The listing builds one solid part. Answer for the finished solid, in the listing's coordinates (mm). Round coordinates to 2 decimals unless told otherwise and drop trailing zeros. Write each loop counter-clockwise with the first axis right and the second up, starting at its lowest first coordinate (ties: lowest second). Pieces come first, ordered by that corner, then holes.
(1) A cutting plane is placed at D-D, the plane x = -80. Give the vertices of the cut face in (y, z).
(2) A cutting plane is placed at A-A, the plane z = 0. Give the vertices of the cut face in (x, y), and give its area (3 significant figures).
(3) Find the intervals of material crossed by probe 1 along Z at (x, y) = (0, -6.5); probe 2 along X at (y, z) = (-7.75, -40); probe 3 along Z at (x, y) = (-40, -4), in increasing order.
(4) This flat-tipped pin is pushed along its axis until it touches: pin 1 Ø10.5 at (x, z) = (-80, 0) entering from +Y. Where does it stop, or does it pass through?
(5) A cutting plane is placed at C-C, the plane z = 40. Give the vertices of the cut face in (x, y).
(6) A cutting plane is placed at B-B, the plane x = 0. Give the vertices of the cut face in (y, z), and give its area (3 significant figures).
from build123d import *

# Parameters (mm, degrees)
BASE_FLANGE1_START     = -75
BASE_FLANGE1_OUTLINE_W = 300
BASE_FLANGE1_OUTLINE_H = 12.7
BASE_FLANGE1_DEPTH     = 150
M10_CLEARANCE_HOLE1_D  = 11
M8_CLEARANCE_HOLE1_D   = 9
CHAMFER1_SIZE          = 10


# Read off the part's stored shape, not the designer's step: Base-Flange1
with BuildPart() as part:
    # Base-Flange1 outline → Base-Flange1 (new body)
    with BuildSketch(Plane.XY.offset(BASE_FLANGE1_START)):
        with Locations((0, -6.35)):
            Rectangle(BASE_FLANGE1_OUTLINE_W, BASE_FLANGE1_OUTLINE_H)
    extrude(amount=BASE_FLANGE1_DEPTH)

    # M10 Clearance Hole1 (through all)
    with Locations(Plane(origin=(0, 0, 0), x_dir=(1, 0, 0), z_dir=(0, 1, 0))):
        with Locations((0, 0)):
            Hole(M10_CLEARANCE_HOLE1_D / 2)

    # M8 Clearance Hole1 (through all)
    with Locations(Plane(origin=(0, 0, 0), x_dir=(1, 0, 0), z_dir=(0, 1, 0))):
        with Locations((-40, 0), (0, -40), (0, 40), (-80, 0)):
            Hole(M8_CLEARANCE_HOLE1_D / 2)

    # Chamfer1
    chamfer1_edges = [part.edges().sort_by_distance(p)[0] for p in [
        (-150, -6.35, 75),
        (-150, -6.35, -75),
        (150, -6.35, -75),
        (150, -6.35, 75),
    ]]
    chamfer(chamfer1_edges, length=CHAMFER1_SIZE)


solid = part.part
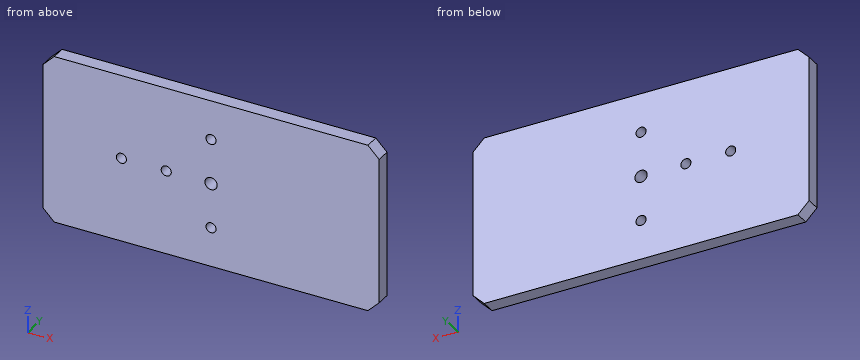
Solutions:
1. outline: (-12.7, -75) - (0, -75) - (0, -4.5) - (-12.7, -4.5) - close; (-12.7, 4.5) - (0, 4.5) - (0, 75) - (-12.7, 75) - close
2. outline: (-150, -12.7) - (-84.5, -12.7) - (-84.5, 0) - (-150, 0) - close; (-75.5, -12.7) - (-44.5, -12.7) - (-44.5, 0) - (-75.5, 0) - close; (-35.5, -12.7) - (-5.5, -12.7) - (-5.5, 0) - (-35.5, 0) - close; (5.5, -12.7) - (150, -12.7) - (150, 0) - (5.5, 0) - close
2. area: 3,440 mm2
3. probe 1: z = -75 to -44.5, -35.5 to -5.5, 5.5 to 35.5, 44.5 to 75
3. probe 2: x = -150 to -4.5, 4.5 to 150
3. probe 3: z = -75 to -4.5, 4.5 to 75
4. pin 1: stops at y = 0
5. outline: (-150, -12.7) - (-4.5, -12.7) - (-4.5, 0) - (-150, 0) - close; (4.5, -12.7) - (150, -12.7) - (150, 0) - (4.5, 0) - close
6. outline: (-12.7, -75) - (0, -75) - (0, -44.5) - (-12.7, -44.5) - close; (-12.7, -35.5) - (0, -35.5) - (0, -5.5) - (-12.7, -5.5) - close; (-12.7, 5.5) - (0, 5.5) - (0, 35.5) - (-12.7, 35.5) - close; (-12.7, 44.5) - (0, 44.5) - (0, 75) - (-12.7, 75) - close
6. area: 1,540 mm2
